from build123d import *

# Parameters (mm, degrees)
SKETCH1_W           = 324.5
SKETCH1_H           = 394
BOSS_EXTRUDE1_DEPTH = 5
SKETCH2_R           = 2.5
CUT_EXTRUDE1_DEPTH  = 256.262732298
SKETCH3_R           = 2.5
CUT_EXTRUDE2_DEPTH  = 5
SKETCH4_R           = 15
SKETCH4_R_2         = 5
CUT_EXTRUDE4_DEPTH  = 256.262732298


with BuildPart() as part:
    # Sketch1 → Boss-Extrude1 (new body)
    with BuildSketch(Plane(origin=(0, 0, 0), x_dir=(1, 0, 0), z_dir=(0, 1, 0))):
        Rectangle(SKETCH1_W, SKETCH1_H)
    extrude(amount=BOSS_EXTRUDE1_DEPTH)

    # Sketch2 → Cut-Extrude1 (cut, through all)
    with BuildSketch(Plane(origin=(0, 5, 0), x_dir=(1, 0, 0), z_dir=(0, 1, 0))):
        with Locations(Location((152.25, 187, 0), (0, 0, 270))):
            Circle(SKETCH2_R)
        with Locations(Location((-152.25, 187, 0), (0, 0, 270))):
            Circle(SKETCH2_R)
        with Locations(Location((-152.25, -187, 0), (0, 0, 270))):
            Circle(SKETCH2_R)
        with Locations(Location((152.25, -187, 0), (0, 0, 270))):
            Circle(SKETCH2_R)
    extrude(amount=-CUT_EXTRUDE1_DEPTH, mode=Mode.SUBTRACT)

    # Sketch3 → Cut-Extrude2 (cut)
    with BuildSketch(Plane(origin=(0, 5, 0), x_dir=(1, 0, 0), z_dir=(0, 1, 0))):
        with Locations(Location((132.25, 0, 0), (0, 0, 270))):
            Circle(SKETCH3_R)
        with Locations(Location((109.75, -38.97114317, 0), (0, 0, 270))):
            Circle(SKETCH3_R)
        with Locations(Location((64.75, -38.97114317, 0), (0, 0, 270))):
            Circle(SKETCH3_R)
        with Locations(Location((42.25, 0, 0), (0, 0, 270))):
            Circle(SKETCH3_R)
        with Locations(Location((64.75, 38.97114317, 0), (0, 0, 270))):
            Circle(SKETCH3_R)
        with Locations(Location((109.75, 38.97114317, 0), (0, 0, 270))):
            Circle(SKETCH3_R)
    extrude(amount=-CUT_EXTRUDE2_DEPTH, mode=Mode.SUBTRACT)

    # Sketch4 → Cut-Extrude4 (cut, through all)
    with BuildSketch(Plane(origin=(0, 5, 0), x_dir=(1, 0, 0), z_dir=(0, 1, 0))):
        with Locations(Location((-109.31, 167, 0), (0, 0, 270))):
            Circle(SKETCH4_R)
        with Locations(Location((-109.31, -167, 0), (0, 0, 270))):
            Circle(SKETCH4_R)
        with Locations(Location((-109.31, 189.5, 0), (0, 0, 270))):
            Circle(SKETCH4_R_2)
        with Locations(Location((-109.31, -189.5, 0), (0, 0, 270))):
            Circle(SKETCH4_R_2)
        with Locations(Location((-131.81, -167, 0), (0, 0, 270))):
            Circle(SKETCH4_R_2)
        with Locations(Location((-109.31, -144.5, 0), (0, 0, 270))):
            Circle(SKETCH4_R_2)
        with Locations(Location((-86.81, -167, 0), (0, 0, 270))):
            Circle(SKETCH4_R_2)
        with Locations(Location((-86.81, 167, 0), (0, 0, 270))):
            Circle(SKETCH4_R_2)
        with Locations(Location((-109.31, 144.5, 0), (0, 0, 270))):
            Circle(SKETCH4_R_2)
        with Locations(Location((-131.81, 167, 0), (0, 0, 270))):
            Circle(SKETCH4_R_2)
    extrude(amount=-CUT_EXTRUDE4_DEPTH, mode=Mode.SUBTRACT)


solid = part.part
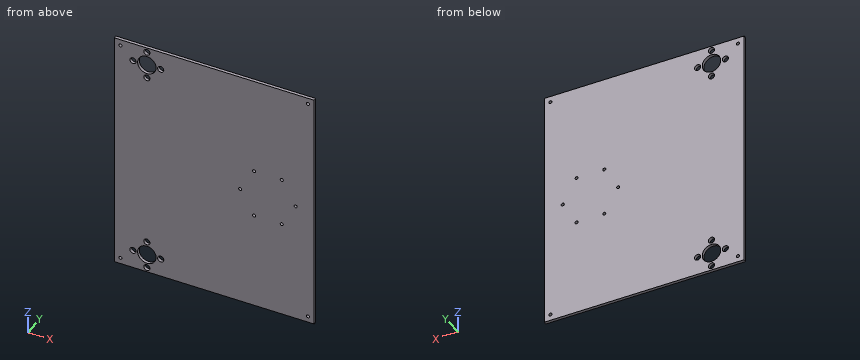
The model under review builds one solid part; all positions refer to its coordinate system, in mm. Coordinates: 2 decimals unless noted, no trailing zeros. Loops run counter-clockwise (first coordinate to the right, second up) from the corner with the lowest first, then second, coordinate; pieces in that order, holes last. Notation, with made-up numbers: M 74,-22.75 L 118,-22.75 A16 ccw 118,7.25 Z; hole C 9.25,39 d4. An arc over 180 degrees is marked long. Put each result on its own line as item: value. Start each with the question number.
Q1. Clearance check with a flat-ended pin moving along its axis: pin 1 (8 mm diameter, centred on x = -131.81, z = 167, fed in from -Y). State where the tip first meets the part, or that it passes through.
Q2. Add section B-B (y = 3.45). Count the separate pieces of the cut face and the enclosed holes in it, and give its area (3 significant figures).
Q3. Add section C-C (x = -131.81). Write out the cut boundary in (y, z).
Q4. Wall thickness on line 1 (X direction, y = 2.25, z = 0); line 2 (Z direction, x = -131, y = 0.95); line 3 (X direction, y = 2.7, z = 144.5): over which ranges is each line inside the solid? List them lowest first.
Q5. Add section A-A (z = 144.5). Write out the cut boundary in (x, y), and give its area (3 significant figures).
Answers:
1. pin 1: passes through
2. separate pieces: 1
2. enclosed holes: 20
2. area: 126,000 mm^2
3. outline: M 0,-197 L 5,-197 L 5,-172 L 0,-172 Z; M 0,-162 L 5,-162 L 5,162 L 0,162 Z; M 0,172 L 5,172 L 5,197 L 0,197 Z
4. line 1: x = -162.25 to 39.75, 44.75 to 129.75, 134.75 to 162.25
4. line 2: z = -197 to -171.93, -162.07 to 162.07, 171.93 to 197
4. line 3: x = -162.25 to -114.31, -104.31 to 162.25
5. outline: M -162.25,0 L -114.31,0 L -114.31,5 L -162.25,5 Z; M -104.31,0 L 162.25,0 L 162.25,5 L -104.31,5 Z
5. area: 1,570 mm^2
